For this review, take the finished solid that the model builds, in its own axes (mm). Face numbers are marked on the shaded views. A direction names the side the tool comes from. Round coordinates to 2 decimals unless told otherwise and drop trailing zeros. Order: outer loops, then holes, each group sorted by start corner. A loop starts at its lowest first (then second) coordinate and runs counter-clockwise, first axis right, second up. Notation, with made-up numbers: (19.25, 37.25) -> (32.25, 37.25) arc R9 cw to (32.25, 47.25) -> close; hole circle Ø2 at (87, 2.5). An arc over 180 degrees is marked (long way). Use a Markdown table: item, result. Add a question column.
1) Consider section D-D (y = 2.75). State the section outline as (x, z) points, plus the area to 3 significant figures.
2) Wall thickness on line 1 along X through (y, z) = (14.75, -35); line 2 along Z through (x, y) = (22, 17); line 3 along Y through (x, z) = (38.5, -14.5): over which ranges is each line inside the solid? List them lowest first. Write a range as [from, to].
3) Consider section C-C (x = 20). State the section outline as (y, z) points.
4) Draft analysis for pull direction X (two halves, no side actions). For the marked faces 3, 4 and 5, state which applies: pulls with the +X half, pulls with the -X half, needs draft (parallel to the pull), parting line crosses it, or undercut.
5) Consider section A-A (z = -36.5). State the section outline as (x, y) points, plus the area to 3 significant figures.
6) Machinability: for the marked faces 1 and 2, which of the approach directions +Z, -Z, +X, -X, +Y, -Y give a long, thin tool a straight path to every point of the face, cutting with its end or side? Answer none if there is none.
7) Clearance check with flat-ended pins moving along their axes: P1, Ø1.5, axis at x = -16.5, z = -21, coming from the +Y side; P2, Ø1.3, axis at x = 14, z = 43.5, coming from the -Y side. State where each tip first meets the part, or that it passes through.
8) Consider section B-B (y = 17.5). State the section outline as (x, z) points, plus the area to 3 significant figures.
Autodesk Inventor part; units mm, degrees
ref_plane "YZ Plane" through (0, 0, 0) normal (1, 0, 0) x (0, 1, 0)
ref_plane "XZ Plane" through (0, 0, 0) normal (0, 1, 0) x (-1, 0, 0)
ref_plane "XY Plane" through (0, 0, 0) normal (0, 0, 1) x (1, 0, 0)
sketch "Sketch1" plane through (0, 0, 0) normal (0, 1, 0) x (-1, 0, 0)
  line L0 (28.1728, 44.1076) -> (-61.8272, 44.1076)
  line L1 (-61.8272, 44.1076) -> (-61.8272, -45.8924)
  line L2 (-61.8272, -45.8924) -> (28.1728, -45.8924)
  line L3 (28.1728, -45.8924) -> (28.1728, 44.1076)
  point P0 (0, 0)
  dimension "d0" = 90
  dimension "d1" = 90
extrude "Extrusion1" add sketch "Sketch1" along normal blind 20
sketch "Sketch2" plane through (0, 20, 0) normal (0, 1, 0) x (1, 0, 0)
  line L0 (-26.9728, -42.9076) -> (60.6272, -42.9076)
  line L1 (60.6272, -42.9076) -> (60.6272, 44.6924)
  line L2 (60.6272, 44.6924) -> (-26.9728, 44.6924)
  line L3 (-26.9728, 44.6924) -> (-26.9728, -42.9076)
  line L4 (-28.1728, 45.8924) -> (-28.1728, -44.1076)
  line L5 (61.8272, 45.8924) -> (-28.1728, 45.8924)
  line L6 (61.8272, -44.1076) -> (61.8272, 45.8924)
  line L7 (-28.1728, -44.1076) -> (61.8272, -44.1076)
  point P0 (0, 0)
  dimension "d4" = 1.2
  dimension "d5" = 1.2
  dimension "d6" = 1.2
  dimension "d7" = 1.2
extrude "Extrusion2" cut sketch "Sketch2" against normal blind 18.8 contours L3 L2 L1 L0
sketch "Sketch3" plane through (-28.1728, 0, 44.1076) normal (0, 0, 1) x (1, 0, 0)
  line L0 (35, 4) -> (55, 4)
  line L1 (55, 4) -> (55, 0)
  line L2 (55, 0) -> (35, 0)
  line L3 (35, 0) -> (35, 4)
  line L4 (0, 0) -> (90, 0)
  line L5 (90, 0) -> (90, 20)
  point P0 (28.1728, 0)
  dimension "d10" = 20
  dimension "d11" = 4
  dimension "d12" = 35
extrude "Extrusion3" cut sketch "Sketch3" against normal blind 90
equation "\"d5\" = d4"
equation "\"d6\" = d4"
equation "\"d7\" = d4"
equation "\"d8\" = d2 - d4"
equation "\"d12\" = -0.5 * d10 + 0.5 * d0"
equation "\"d13\" = d0"
properties part number "weight_holder"
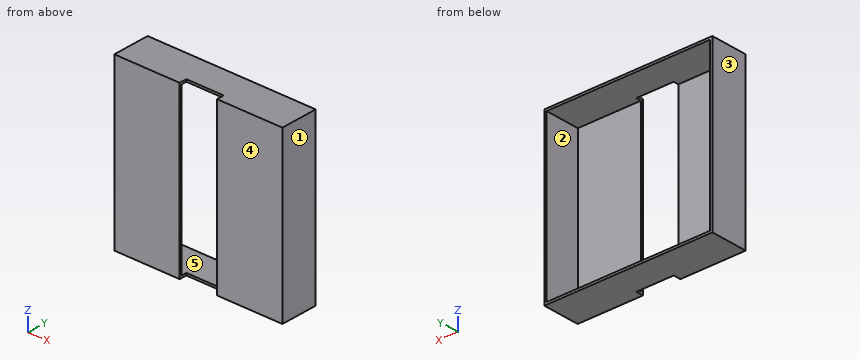
Results list:
| question | item | result |
|---|---|---|
| 1 | outline | (-28.17, -45.89) -> (6.83, -45.89) -> (6.83, -44.69) -> (-26.97, -44.69) -> (-26.97, 42.91) -> (6.83, 42.91) -> (6.83, 44.11) -> (-28.17, 44.11) -> close; (26.83, -45.89) -> (61.83, -45.89) -> (61.83, 44.11) -> (26.83, 44.11) -> (26.83, 42.91) -> (60.63, 42.91) -> (60.63, -44.69) -> (26.83, -44.69) -> close |
| 1 | area | 378 mm2 |
| 2 | line 1 | [-28.17, -26.97], [60.63, 61.83] |
| 2 | line 2 | [-45.89, -44.69], [42.91, 44.11] |
| 2 | line 3 | [0, 1.2] |
| 3 | outline | (4, -45.89) -> (20, -45.89) -> (20, -44.69) -> (4, -44.69) -> close; (4, 42.91) -> (20, 42.91) -> (20, 44.11) -> (4, 44.11) -> close |
| 4 | face 3 | pulls with the -X half |
| 4 | face 4 | needs draft |
| 4 | face 5 | undercut |
| 5 | outline | (-28.17, 0) -> (6.83, 0) -> (6.83, 1.2) -> (-26.97, 1.2) -> (-26.97, 20) -> (-28.17, 20) -> close; (26.83, 0) -> (61.83, 0) -> (61.83, 20) -> (60.63, 20) -> (60.63, 1.2) -> (26.83, 1.2) -> close |
| 5 | area | 129 mm2 |
| 6 | face 1 | +Z, -Z, +X, +Y, -Y |
| 6 | face 2 | +Y |
| 7 | P1 | y = 1.2 |
| 7 | P2 | y = 4 |
| 8 | outline | (-28.17, -45.89) -> (61.83, -45.89) -> (61.83, 44.11) -> (-28.17, 44.11) -> close; hole (-26.97, -44.69) -> (60.63, -44.69) -> (60.63, 42.91) -> (-26.97, 42.91) -> close |
| 8 | area | 426 mm2 |
